Part model, mm, in its own coordinate system. A direction names the side the tool comes from. Give positions to 0.01 mm unless a question says otherwise; leave off trailing zeros. Order: outer loops, then holes, each group sorted by start corner. A loop starts at its lowest first (then second) coordinate and runs counter-clockwise, first axis right, second up. Notation, with made-up numbers: (49, 30) - (83, 30) arc R8 ccw to (83, 34) - close; hole circle Ø2 at (55, 9). An arc over 180 degrees is marked (long way). Use one line per item in the form item = value. Start each with the question number.
1. Band-saw the part on A-A, the plane x = 0. List the corners of the cut face in (y, z).
2. Pull direction Z, two halves, no side cores. Call faces 6 (the face through (11.976, 0.174, -44.956)), 7 (the face through (-6, 0, 0)), 8 (the face through (-27.811, -14.276, -3.541)), 9 (the face through (-6.477, -2.04, -23.881)): +Z half, -Z half, draft (parallel to the pull), parting line (faces both ways), or undercut.
3. Pin check, flat tips, straight feed: P1, Ø11, axis at x = -1.5, y = 0.5, coming from the -Z side; P2, Ø12.5, axis at y = 6, z = -27, coming from the -X side; P3, Ø4, axis at x = -18, y = -2.5, coming from the -Z side (3 decimals). Stop position of each tip, or through.
4. Band-saw the part on B-B, the plane z = -41. List the corners of the cut face in (x, y), plus the area to 3 significant figures.
5. Tool access for faces 1 (the face through (20.562, -14.276, -8.761)), 2 (the face through (12.7, 0, -27)), 3 (the face through (11.976, 14.236, -27.84)), 4 (the face through (-20.713, 14.276, -8.761)), 5 (the face through (-11.936, -14.276, -27.84)): list every direction of +Z, -Z, +X, -X, +Y, -Y with a clear straight run to the whole face (end or side of a thin tool).
6. Band-saw the part on C-C, the plane y = 9. List the corners of the cut face in (x, z) (3 decimals), plus the area to 3 significant figures.
7. Drill centre lines: line 1 (Y direction, x = 0, z = -25); line 2 (X direction, y = 8.75, z = -39.5); line 3 (X direction, y = 1.5, z = -7). Where is each one in solid material? Low to high.
8. Band-saw the part on D-D, the plane y = 0. State how many separate pieces and enclosed holes the cut face has, plus the area to 3 significant figures.
from build123d import *

# Parameters (mm, degrees)
SKETCH3_W              = 57.15
SKETCH3_H              = 30
SKETCH3_R              = 12.7
BOSS_EXTRUDE1_DEPTH    = 9.525
SKETCH6_W              = 25.4
SKETCH6_H              = 30
SKETCH6_R              = 11.684
BOSS_EXTRUDE2_DEPTH    = 36.195
F_10_CLEARANCE_HOLE1_D = 4.9784
FILLET2_R              = 2.54


with BuildPart() as part:
    # Sketch1 → Revolve1 (revolve)
    with BuildSketch(Plane(origin=(0, 0, 0), x_dir=(1, 0, 0), z_dir=(0, 1, 0)), mode=Mode.PRIVATE) as revolve1_sk:
        Polygon((4.80625, 6.35), (4.80625, 0), (12.7, 0), (12.7, 45.72), (4.7625, 45.72), (4.7625, 41.91), (6.790625, 41.91), (6.790625, 6.35), align=None)
    revolve(revolve1_sk.sketch.rotate(Axis((0, 0, 0), (0, 0, 1)), 180), axis=Axis((0, 0, 0), (0, 0, 1)))  # turned: the seam where the file's is

    # Sketch3 → Boss-Extrude1 (add)
    with BuildSketch(Plane(origin=(0, 0, 0), x_dir=(-1, 0, 0), z_dir=(0, 0, -1))):
        Rectangle(SKETCH3_W, SKETCH3_H)
        Circle(SKETCH3_R, mode=Mode.SUBTRACT)
    extrude(amount=BOSS_EXTRUDE1_DEPTH)

    # Sketch6 → Boss-Extrude2 (add)
    with BuildSketch(Plane(origin=(0, 0, -9.525), x_dir=(-1, 0, 0), z_dir=(0, 0, -1))):
        Rectangle(SKETCH6_W, SKETCH6_H)
        Circle(SKETCH6_R, mode=Mode.SUBTRACT)
    extrude(amount=BOSS_EXTRUDE2_DEPTH)

    # #10 Clearance Hole1 (through all)
    with Locations(Plane(origin=(0, 0, -9.525), x_dir=(-1, 0, 0), z_dir=(0, 0, -1))):
        with Locations((20.6375, 0), (-20.6375, 0)):
            Hole(F_10_CLEARANCE_HOLE1_D / 2)

    # Fillet2
    fillet2_edges = [part.edges().sort_by_distance(p)[0] for p in [
        (28.575, 0, -9.525),
        (20.6375, -15, -9.525),
        (-28.575, 0, -9.525),
        (-20.6375, 15, -9.525),
        (28.575, 15, -4.7625),
        (28.575, -15, -4.7625),
        (-28.575, -15, -4.7625),
        (-28.575, 15, -4.7625),
        (20.6375, 15, -9.525),
        (-20.6375, -15, -9.525),
        (12.7, 0, -9.525),
        (12.7, 0, -45.72),
        (12.7, 15, -27.6225),
        (-12.7, 0, -9.525),
        (-12.7, 0, -45.72),
        (-12.7, -15, -27.6225),
        (0, -15, -45.72),
        (12.7, -15, -27.6225),
        (0, 15, -45.72),
        (-12.7, 15, -27.6225),
        (4.7625, 0, -45.72),
    ]]
    fillet(fillet2_edges, radius=FILLET2_R)


solid = part.part
From the geometry:
q1.outline = (-15, -43.18) arc R2.54 ccw to (-12.46, -45.72) - (-7.3, -45.72) arc R2.54 ccw to (-4.76, -43.18) - (-4.76, -41.91) - (-6.79, -41.91) - (-6.79, -6.35) - (-4.81, -6.35) - (-4.81, 0) - (-15, 0) - close; (4.76, -43.18) arc R2.54 ccw to (7.3, -45.72) - (12.46, -45.72) arc R2.54 ccw to (15, -43.18) - (15, 0) - (4.81, 0) - (4.81, -6.35) - (6.79, -6.35) - (6.79, -41.91) - (4.76, -41.91) - close
q2.face_6 = -Z half
q2.face_7 = +Z half
q2.face_8 = draft
q2.face_9 = undercut
q3.P1 = -45.71
q3.P2 = -12.7
q3.P3 = -9.525
q4.outline = (-12.7, -12.46) arc R2.54 ccw to (-10.16, -15) - (10.16, -15) arc R2.54 ccw to (12.7, -12.46) - (12.7, 12.46) arc R2.54 ccw to (10.16, 15) - (-10.16, 15) arc R2.54 ccw to (-12.7, 12.46) - close; hole circle Ø13.58 at (0, 0)
q4.area = 612 mm²
q5.face_1 = -Z, +X, -Y
q5.face_2 = -Z, +X, +Y, -Y
q5.face_3 = -Z, +X, +Y
q5.face_4 = -Z, -X, +Y
q5.face_5 = -Z, -X, -Y
q6.outline = (-28.575, -6.985) arc R2.54 ccw to (-26.035, -9.525) - (-15.24, -9.525) arc R2.54 cw to (-12.7, -12.065) - (-12.7, -43.18) arc R2.54 ccw to (-10.16, -45.72) - (10.16, -45.72) arc R2.54 ccw to (12.7, -43.18) - (12.7, -12.065) arc R2.54 cw to (15.24, -9.525) - (26.035, -9.525) arc R2.54 ccw to (28.575, -6.985) - (28.575, 0) - (-28.575, 0) - close
q6.area = 1,460 mm²
q7.line_1 = -15 to -6.79, 6.79 to 15
q7.line_2 = -12.7 to 12.7
q7.line_3 = -28.57 to -22.62, -18.65 to -6.62, 6.62 to 18.65, 22.62 to 28.57
q8.separate_pieces = 4
q8.enclosed_holes = 0
q8.area = 783 mm²
